```python
from build123d import *

# Parameters (mm, degrees)
SKETCH_1_R      = 2.5
EXTRUDE_1_DEPTH = 34
EXTRUDE_2_DEPTH = 6
EXTRUDE_START   = 6
EXTRUDE_3_DEPTH = 6


with BuildPart() as part:
    # 草图1 → 凸台-拉伸1 (new body)
    with BuildSketch(Plane(origin=(0, 0, 0), x_dir=(1, 0, 0), z_dir=(0, 1, 0))):
        with Locations(Location((0, 0, 0), (0, 0, 270))):
            Circle(SKETCH_1_R)
    extrude(amount=EXTRUDE_1_DEPTH)

    # 草图2 → 凸台-拉伸2 (add)
    with BuildSketch(Plane(origin=(0, 34, 0), x_dir=(1, 0, 0), z_dir=(0, 1, 0))):
        with BuildLine():
            Line((1, 1.118033989), (1, -1.118033989))
            ThreePointArc((1, -1.118033989), (-1.5, 0), (1, 1.118033989))
        make_face()
    extrude(amount=EXTRUDE_2_DEPTH)

    # 草图3 → 凸台-拉伸3 (add)
    with BuildSketch(Plane.XZ.offset(EXTRUDE_START)):
        with BuildLine():
            Line((1, -1.118033989), (1, 1.118033989))
            ThreePointArc((1, 1.118033989), (-1.5, 0), (1, -1.118033989))
        make_face()
    extrude(amount=-EXTRUDE_3_DEPTH)


solid = part.part
```
Input: part model. Units: mm. Frame: model coordinates. A direction names the side the tool comes from. Give positions to 0.01 mm unless a question says otherwise; leave off trailing zeros. Order: outer loops, then holes, each group sorted by start corner. A loop starts at its lowest first (then second) coordinate and runs counter-clockwise, first axis right, second up. Notation, with made-up numbers: M -26.5,59 L 10.5,59 A24 ccw 10.5,92 Z; hole C 15.25,88.25 d2. An arc over 180 degrees is marked long. One line per question, with ' | ' between items. Start each with the question number.
1. Material intervals for probe 1 along Y at (x, z) = (-0.95, 1.5); probe 2 along Z at (x, y) = (2, 27.5); probe 3 along Z at (x, y) = (1.15, 2.5), sorted ascending. Write a range as [from, to].
2. First-contact query: pin 1 Ø0.7 at (y, z) = (-3.5, 0) entering from +X. Flat tip, straight axial feed; report the tip coordinate or a pass-through.
3. Access query for faces 1 (the face through (1, -3, 0)), 2 (the face through (-1.5, 37, 0)), 3 (the face through (-1.5, -3, 0)), 4 (the face through (1, 37, 0)), 5 (the face through (0, -6, 0)). Directions: +Z, -Z, +X, -X, +Y, -Y. A direction counts if a zero-diameter tool reaches every point of the face in a straight line with its end or side. Return the directions, or none.
4. Section query A-A (z = 0). Return the cut outline in (x, y), and give its area (3 significant figures).
5. Section query B-B (x = 0). Return the cut outline in (y, z).
6. Section query C-C (y = 3). Return the cut outline in (x, z), and give its area (3 significant figures).
Here are the results:
1) probe 1: [0, 34] | probe 2: [-1.5, 1.5] | probe 3: [-2.22, 2.22]
2) pin 1: x = 1
3) face 1: +Z, -Z, +X, -Y | face 2: +Y | face 3: -Y | face 4: +Z, -Z, +X, +Y | face 5: +Z, -Z, +X, -X, -Y
4) outline: M -2.5,0 L -1.5,0 L -1.5,-6 L 1,-6 L 1,0 L 2.5,0 L 2.5,34 L 1,34 L 1,40 L -1.5,40 L -1.5,34 L -2.5,34 Z | area: 200 mm²
5) outline: M -6,-1.5 L 0,-1.5 L 0,-2.5 L 34,-2.5 L 34,-1.5 L 40,-1.5 L 40,1.5 L 34,1.5 L 34,2.5 L 0,2.5 L 0,1.5 L -6,1.5 Z
6) outline: C 0,0 d5 | area: 19.6 mm²
